from build123d import *

# Parameters (mm, degrees)
CROQUIS1_R              = 9.75
SALIENTE_EXTRUIR1_DEPTH = 3
CROQUIS2_R              = 1.25
CORTAR_EXTRUIR1_DEPTH   = 3


with BuildPart() as part:
    # Croquis1 → Saliente-Extruir1 (new body)
    with BuildSketch(Plane.XY):
        with BuildLine():
            Line((-14, -25), (14, -25))
            Line((14, -25), (14, 0))
            ThreePointArc((14, 0), (0, 14), (-14, 0))
            Line((-14, 0), (-14, -25))
        make_face()
        Circle(CROQUIS1_R, mode=Mode.SUBTRACT)
    extrude(amount=SALIENTE_EXTRUIR1_DEPTH)

    # Croquis2 → Cortar-Extruir1 (cut)
    with BuildSketch(Plane.XY.offset(3)):
        with Locations((0, -19.5)):
            Circle(CROQUIS2_R)
        with Locations((7.5, -19.5)):
            Circle(CROQUIS2_R)
        with Locations((-7.5, -19.5)):
            Circle(CROQUIS2_R)
    extrude(amount=-CORTAR_EXTRUIR1_DEPTH, mode=Mode.SUBTRACT)


solid = part.part
Input: part model. Units: mm. Frame: model coordinates. Coordinates: 2 decimals unless noted, no trailing zeros. Loops run counter-clockwise (first coordinate to the right, second up) from the corner with the lowest first, then second, coordinate; pieces in that order, holes last. Notation, with made-up numbers: (-1, 44) -> (32, 44) arc R18 ccw to (32, 66) -> close; hole circle Ø11 at (49, 21). An arc over 180 degrees is marked (long way). Write each question's results on one line, items separated by ' | '. Start each with the question number.
Q1. Section C-C, the plane x = 4.75. Return the cut outline in (y, z), plus the area to 3 significant figures.
Q2. Section D-D, the plane y = 6.5. Return the cut outline in (x, z).
Q3. Section A-A, the plane y = -19.5. Return the cut outline in (x, z).
Q4. Pin query (flat end, axial travel): pin 1 (1 mm diameter, centred on x = -0.5, z = 2.5, fed in from +Y); pin 2 (1 mm diameter, centred on y = 4, z = 1, fed in from +X). Return the tip coordinate at first contact, or that it passes through.
Q5. Ray query, line 1 (Y direction, x = 0, z = 0.85); line 2 (Y direction, x = -7.75, z = 1.5); line 3 (X direction, y = -20, z = 2.4). Return the intervals inside material, ascending. Write a range as from..to.
Q6. Pull-direction query (X, two-part tool) for faces 1 (the flat face through (-14, -12, 1)), 2 (the cylindrical face through (-0.27, -20.72, 1.52)), 3 (the cylindrical face through (0, 14, 1)), 4 (the flat face through (0, -25, 1)); classes: released by +X, released by -X, zero draft, split by the parting line, or undercut.
Q7. Section B-B, the plane z = 1.7. Return the cut outline in (x, y), plus the area to 3 significant figures.
Found:
1) outline: (-25, 0) -> (-8.51, 0) -> (-8.51, 3) -> (-25, 3) -> close; (8.51, 0) -> (13.17, 0) -> (13.17, 3) -> (8.51, 3) -> close | area: 63.4 mm2
2) outline: (-12.4, 0) -> (-7.27, 0) -> (-7.27, 3) -> (-12.4, 3) -> close; (7.27, 0) -> (12.4, 0) -> (12.4, 3) -> (7.27, 3) -> close
3) outline: (-14, 0) -> (-8.75, 0) -> (-8.75, 3) -> (-14, 3) -> close; (-6.25, 0) -> (-1.25, 0) -> (-1.25, 3) -> (-6.25, 3) -> close; (1.25, 0) -> (6.25, 0) -> (6.25, 3) -> (1.25, 3) -> close; (8.75, 0) -> (14, 0) -> (14, 3) -> (8.75, 3) -> close
4) pin 1: y = 14 | pin 2: x = 13.56
5) line 1: -25..-20.75, -18.25..-9.75, 9.75..14 | line 2: -25..-20.72, -18.28..-5.92, 5.92..11.66 | line 3: -14..-8.65, -6.35..-1.15, 1.15..6.35, 8.65..14
6) face 1: released by -X | face 2: undercut | face 3: split by the parting line | face 4: zero draft
7) outline: (-14, -25) -> (14, -25) -> (14, 0) arc R14 ccw to (-14, 0) -> close; hole circle Ø19.5 at (0, 0); hole circle Ø2.5 at (-7.5, -19.5); hole circle Ø2.5 at (0, -19.5); hole circle Ø2.5 at (7.5, -19.5) | area: 695 mm2
